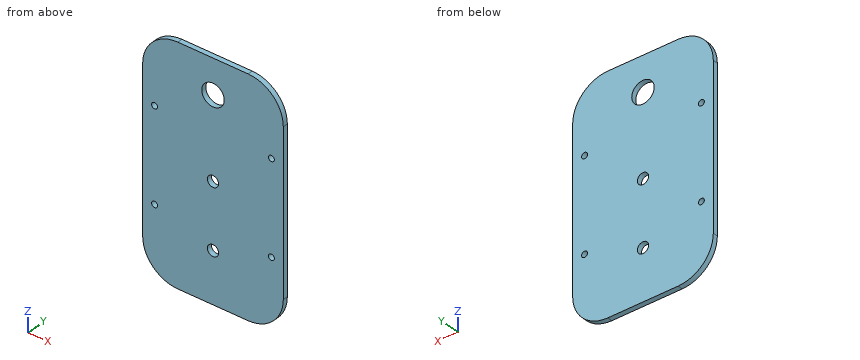
Autodesk Inventor part; units mm, degrees
ref_plane "YZ Plane" through (0, 0, 0) normal (1, 0, 0) x (0, 1, 0)
ref_plane "XZ Plane" through (0, 0, 0) normal (0, 1, 0) x (-1, 0, 0)
ref_plane "XY Plane" through (0, 0, 0) normal (0, 0, 1) x (1, 0, 0)
sketch "Sketch1" plane through (0, 0, 0) normal (0, 1, 0) x (-1, 0, 0)
  line L0 (-75, 125) -> (75, 125)
  line L1 (75, 125) -> (75, -125)
  line L2 (75, -125) -> (-75, -125)
  line L3 (-75, -125) -> (-75, 125)
  line L4 (-75, 125) -> (75, -125) construction
  line L5 (75, 125) -> (-75, -125) construction
  point P0 (0, 0)
  dimension "d0" = 150
  dimension "d1" = 250
extrude "Extrusion1" add sketch "Sketch1" along normal blind 5.4
fillet "Fillet1" radius 37.5 4 edges at (75, 2.7, 125) (75, 2.7, -125) (-75, 2.7, 125) (-75, 2.7, -125)
sketch "Sketch2" plane through (0, 5.4, 0) normal (0, 1, 0) x (1, 0, 0)
  line L0 (37.5, -125) -> (-37.5, -125)
  line L1 (-37.5, -125) -> (-37.5, -50)
  line L2 (-37.5, -50) -> (37.5, -50)
  line L3 (37.5, -50) -> (37.5, -125)
  line L4 (-37.5, -125) -> (37.5, -125)
  line L5 (-75, 87.5) -> (-75, -87.5)
  circle A0 centre (0, -87.5) radius 12
  point P0 (0, 0)
  point P1 (-37.5, -87.5)
  point P2 (0, -50)
  dimension "d6" = 75
  dimension "d7" = 0
  dimension "d9" = 24
  dimension "d10" = 37.5
  dimension "d11" = 37.5
extrude "Extrusion2" cut sketch "Sketch2" against normal blind 20.5 contours A0
sketch "Sketch3" plane through (0, 5.4, 0) normal (0, 1, 0) x (1, 0, 0)
  circle A0 centre (0, 0) radius 6
  circle A1 centre (0, 70) radius 6
  line L0 (37.5, 125) -> (-37.5, 125)
  line L1 (-75, 87.5) -> (-75, -87.5)
  line L2 (-37.5, -125) -> (37.5, -125)
  line L3 (75, -87.5) -> (75, 87.5)
  point P0 (0, 125)
  point P1 (0, 125)
  point P2 (0, -125)
  dimension "d15" = 12
  dimension "d16" = 55
  dimension "d21" = 75
  dimension "d22" = 125
  dimension "d23" = 250
  dimension "d24" = 150
extrude "Extrusion3" cut sketch "Sketch3" against normal blind 40
sketch "Sketch4" plane through (0, 5.4, 0) normal (0, 1, 0) x (1, 0, 0)
  circle A0 centre (-62.3, 50) radius 3.175
  line L0 (37.5, 125) -> (-37.5, 125)
  line L1 (-75, 87.5) -> (-75, -87.5)
  circle A1 centre (-62.3, -50) radius 3.175
  circle A2 centre (62.3, 50) radius 3.175
  circle A3 centre (62.3, -50) radius 3.175
  point P0 (0, 0)
  dimension "d27" = 100
  dimension "d30" = 124.6
  dimension "d33" = 12.7
  dimension "d34" = 6.35
  dimension "d35" = 50
extrude "Extrusion4" cut sketch "Sketch4" against normal blind 40
equation "\"d21\" = 0.5 * d24"
equation "\"d27\" = 2 * d35"
properties part number "Plate"
Can you work these out from the model? Positions are in its coordinate system, mm. Give positions to 0.01 mm unless a question says otherwise; leave off trailing zeros. Write each loop counter-clockwise with the first axis right and the second up, starting at its lowest first coordinate (ties: lowest second). Pieces come first, ordered by that corner, then holes. Notation, with made-up numbers: (-14, 68.5) -> (22, 68.5) arc R32 cw to (22, 107.5) -> close; hole circle Ø2 at (82, 66.5). An arc over 180 degrees is marked (long way). Answer as a JSON object with one key per item and string values. Group by question number.
Item 1: Suppose I cut it at A-A (x = 0). Please give me the cut outline in (y, z), plus the area to 3 significant figures.
Item 2: Suppose I cut it at B-B (y = 1.55). Please give me the cut outline in (x, z) (3 decimals).
Item 3: I'm going to push flat-ended pins straight in: P1, Ø8.5, axis at x = 62.3, z = 50, coming from the +Y side; P2, Ø11, axis at x = 0, z = 0, coming from the +Y side. Where does each tip first touch, or does it pass through?
Item 4: Suppose I cut it at D-D (x = 62.3). Please give me the cut outline in (y, z) (3 decimals), plus the area to 3 significant figures.
Item 5: Suppose I cut it at C-C (z = -50). Please give me the cut outline in (x, y) (3 decimals).
Item 6: Please list where these lines run through material, in increasing order: line 1 (X direction, y = 0.5, z = -50) (3 decimals); line 2 (Z direction, x = 0, y = 1.15); line 3 (Z direction, x = 62.3, y = 4) (3 decimals). Write a range as [from, to].
Findings:
{
 "1": {"outline": "(0, -125) -> (5.4, -125) -> (5.4, -76) -> (0, -76) -> close; (0, -64) -> (5.4, -64) -> (5.4, -6) -> (0, -6) -> close; (0, 6) -> (5.4, 6) -> (5.4, 75.5) -> (0, 75.5) -> close; (0, 99.5) -> (5.4, 99.5) -> (5.4, 125) -> (0, 125) -> close", "area": "1,090 mm²"},
 "2": {"outline": "(-75, -87.5) arc R37.5 ccw to (-37.5, -125) -> (37.5, -125) arc R37.5 ccw to (75, -87.5) -> (75, 87.5) arc R37.5 ccw to (37.5, 125) -> (-37.5, 125) arc R37.5 ccw to (-75, 87.5) -> close; hole circle Ø6.35 at (-62.3, -50); hole circle Ø6.35 at (-62.3, 50); hole circle Ø24 at (0, 87.5); hole circle Ø12 at (0, -70); hole circle Ø12 at (0, 0); hole circle Ø6.35 at (62.3, -50); hole circle Ø6.35 at (62.3, 50)"},
 "3": {"P1": "stops at y = 5.4", "P2": "passes through"},
 "4": {"outline": "(0, -115.628) -> (5.4, -115.628) -> (5.4, -53.175) -> (0, -53.175) -> close; (0, -46.825) -> (5.4, -46.825) -> (5.4, 46.825) -> (0, 46.825) -> close; (0, 53.175) -> (5.4, 53.175) -> (5.4, 115.628) -> (0, 115.628) -> close", "area": "1,180 mm²"},
 "5": {"outline": "(-75, 0) -> (-65.475, 0) -> (-65.475, 5.4) -> (-75, 5.4) -> close; (-59.125, 0) -> (59.125, 0) -> (59.125, 5.4) -> (-59.125, 5.4) -> close; (65.475, 0) -> (75, 0) -> (75, 5.4) -> (65.475, 5.4) -> close"},
 "6": {"line 1": "x = [-75, -65.475], [-59.125, 59.125], [65.475, 75]", "line 2": "z = [-125, -76], [-64, -6], [6, 75.5], [99.5, 125]", "line 3": "z = [-115.628, -53.175], [-46.825, 46.825], [53.175, 115.628]"}
}
